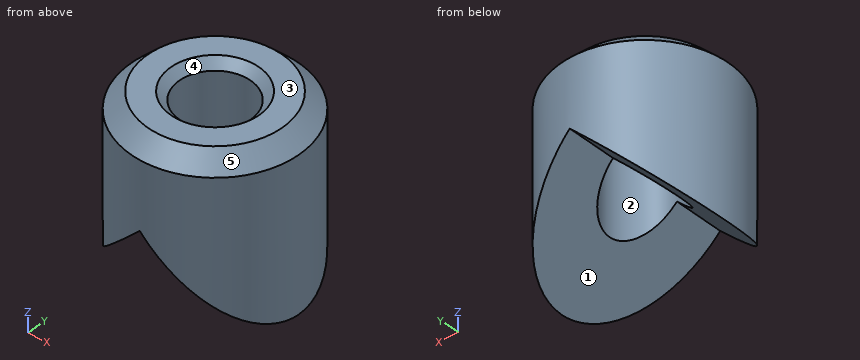
```python
from build123d import *

# Parameters (mm, degrees)
F0_R     = 10
F0_R_2   = 4.25
F1_DEPTH = 20
F3_DEPTH = 12.5
F4_SIZE  = 2
F5_SIZE  = 1


with BuildPart() as f1:
    # F0 (on Top) → F1 (new body)
    with BuildSketch(Plane.XY):
        Circle(F0_R)
        Circle(F0_R_2, mode=Mode.SUBTRACT)
    extrude(amount=F1_DEPTH)

    # F2 (on Front) → F3 (cut, symmetric)
    with BuildSketch(Plane.XZ):
        Polygon((0, 10.010473), (-10.010473, 0), (10.010473, 0), align=None)
    extrude(amount=F3_DEPTH, both=True, mode=Mode.SUBTRACT)

    # F4
    f4_edges = [f1.edges().sort_by_distance(p)[0] for p in [
        (-10, 0, 20),
    ]]
    chamfer(f4_edges, length=F4_SIZE)

    # F5
    f5_edges = [f1.edges().sort_by_distance(p)[0] for p in [
        (-4.25, 0, 20),
    ]]
    chamfer(f5_edges, length=F5_SIZE)


solid = f1.part
```
CAD build for the part. Positions are in the model's coordinates, mm. Face numbers are marked on the shaded views. A direction names the side the tool comes from. Round coordinates to 2 decimals unless told otherwise and drop trailing zeros. Write each loop counter-clockwise with the first axis right and the second up, starting at its lowest first coordinate (ties: lowest second). Pieces come first, ordered by that corner, then holes. Notation, with made-up numbers: (24, 36.5) - (31, 36.5) arc R11 ccw to (31, 47.5) - close; hole circle Ø4 at (66.5, 14.25). An arc over 180 degrees is marked (long way). Return JSON: item names as keys, results as strings. Group by question number.
Item 1: Band-saw the part on C-C on z = 11.5. List the corners of the cut face in (x, y).
Item 2: Mould opens along X. For the marked faces 3, 4 and 5 say: +X half, -X half, draft (parallel to the pull), parting line (faces both ways), or undercut.
Item 3: Band-saw the part on D-D on z = 3.5. List the corners of the cut face in (x, y).
Item 4: 3-axis set-ups, long thin cutter, end or side, ignore diameter. For the marked faces 1 and 2: which of +Z, -Z, +X, -X, +Y, -Y reach the whole face in a straight line?
Item 5: Flat gauge pins, fed straight in: pin 1 Ø1 at (y, z) = (2.5, 3.5) entering from +X; pin 2 Ø4 at (x, y) = (6.5, -1.5) entering from -Z; pin 3 Ø6 at (x, z) = (2, 14.5) entering from +Y; pin 4 Ø2 at (x, y) = (3.5, -2) entering from +Z. Where does each tip first touch, or does it go through?
Item 6: Band-saw the part on B-B on z = 7. List the corners of the cut face in (x, y).
Item 7: Probe probe 1 along X at (y, z) = (0, 12.75); probe 2 along Y at (x, z) = (-1, 11). List the from-to ranges inside material, lowest first.
Item 8: Band-saw the part on A-A on y = 0. List the corners of the cut face in (x, z), plus the area to 3 significant figures.
Resolved:
{
 "1": {"outline": "circle Ø20 at (0, 0); hole circle Ø8.5 at (0, 0)"},
 "2": {"face 3": "draft", "face 4": "undercut", "face 5": "parting line"},
 "3": {"outline": "(-6.51, -7.59) - (-6.51, 7.59) arc R10 ccw to start; (6.51, -7.59) arc R10 ccw to (6.51, 7.59) - close"},
 "4": {"face 1": "-Z, +Y, -Y", "face 2": "+Z, -Z"},
 "5": {"pin 1": "stops at x = 9.8", "pin 2": "stops at z = 1.51", "pin 3": "stops at y = 10", "pin 4": "stops at z = 19.78"},
 "6": {"outline": "(-3.01, -9.54) - (-3.01, -3) arc R4.25 cw to (-3.01, 3) - (-3.01, 9.54) arc R10 ccw to start; (3.01, -9.54) arc R10 ccw to (3.01, 9.54) - (3.01, 3) arc R4.25 cw to (3.01, -3) - close"},
 "7": {"probe 1": "x = -10 to -4.25, 4.25 to 10", "probe 2": "y = -9.95 to -4.13, 4.13 to 9.95"},
 "8": {"outline": "(-10, 0.01) - (-4.25, 5.76) - (-4.25, 19) - (-5.25, 20) - (-8, 20) - (-10, 18) - close; (4.25, 5.76) - (10, 0.01) - (10, 18) - (8, 20) - (5.25, 20) - (4.25, 19) - close", "area": "192 mm²"}
}
